```python
from build123d import *

# Parameters (mm, degrees)
BOSS_EXTRUDE1_DEPTH = 15
SKETCH4_R           = 1.5875
CUT_EXTRUDE2_DEPTH  = 25.005207768
SKETCH6_W           = 7.103151839
SKETCH6_H           = 13
SKETCH6_W_2         = 1.996848161
BOSS_EXTRUDE2_DEPTH = 8
SKETCH7_W           = 5.475
SKETCH7_H           = 24
CUT_EXTRUDE3_DEPTH  = 30.261749777


with BuildPart() as part:
    # Sketch1 → Boss-Extrude1 (new body)
    with BuildSketch(Plane(origin=(0, 0, 0), x_dir=(0, 0, -1), z_dir=(1, 0, 0))):
        with BuildLine():
            Line((6.5, 0), (13.5, 0))
            Line((13.5, 0), (13.5, -13))
            Line((13.5, -13), (-13.5, -13))
            Line((-13.5, -13), (-13.5, 0))
            Line((-13.5, 0), (-6.5, 0))
            ThreePointArc((-6.5, 0), (0, -6.5), (6.5, 0))
        make_face()
    extrude(amount=BOSS_EXTRUDE1_DEPTH)

    # Sketch4 → Cut-Extrude2 (cut, through all)
    with BuildSketch(Plane.XZ.offset(13)):
        with Locations(Location((10.2375, -10.75, 0), (0, 0, 270))):
            Circle(SKETCH4_R)
        with Locations(Location((10.2375, 10.75, 0), (0, 0, 270))):
            Circle(SKETCH4_R)
    extrude(amount=-CUT_EXTRUDE2_DEPTH, mode=Mode.SUBTRACT)

    # Sketch6 → Boss-Extrude2 (add)
    with BuildSketch(Plane.XY.offset(13.5)):
        with Locations((11.448424081, -6.5)):
            Rectangle(SKETCH6_W, SKETCH6_H)
        with Locations((0.998424081, -6.5)):
            Rectangle(SKETCH6_W_2, SKETCH6_H)
    extrude(amount=BOSS_EXTRUDE2_DEPTH)

    # Sketch7 → Cut-Extrude3 (cut, through all)
    with BuildSketch(Plane(origin=(0, 0, 0), x_dir=(1, 0, 0), z_dir=(0, 1, 0))):
        with Locations((2.7375, 1.5)):
            Rectangle(SKETCH7_W, SKETCH7_H)
    extrude(amount=-CUT_EXTRUDE3_DEPTH, mode=Mode.SUBTRACT)


solid = part.part
```
Part model, mm, in its own coordinate system. A direction names the side the tool comes from. Round coordinates to 2 decimals unless told otherwise and drop trailing zeros. Loops run counter-clockwise (first coordinate to the right, second up) from the corner with the lowest first, then second, coordinate; pieces in that order, holes last. Notation, with made-up numbers: (-36.75, -35) -> (-0.75, -35) arc R23 cw to (-0.75, 4) -> close; hole circle Ø4 at (-40, 85). An arc over 180 degrees is marked (long way). Use CSV: the item, a comma, the result in double quotes. Start each with the question number.
1) Which spindle directions (+Z, -Z, +X, -X, +Y, -Y) get a long thin tool onto all of the face, cutting with end or side? Do faces 1 (the cylindrical face through (10.2, -6.5, 0.1)), 2 (the flat face through (7.897, -7, 17)), 3 (the flat face through (3, -6, 10.5)). Say none if no direction does.
2) Drop flat-ended pins along their axis: P1, Ø6.5, axis at y = -4.5, z = -1.5, coming from the -X side (3 decimals); P2, Ø2.5, axis at x = 10.24, z = 10.75, coming from the -Y side. Give the stop position or say it passes through.
3) Cut at A-A, the plane z = 14.5. Write the cut outline in (x, y).
4) Pull direction Z, two halves, no side cores. Call faces 4 (the cylindrical face through (11.81, -6.59, -10.54)), 5 (the flat face through (5, -7, 13.5)), 6 (the flat face through (11, 0, -9)): +Z half, -Z half, draft (parallel to the pull), parting line (faces both ways), or undercut.
5) Wall check: L1, parallel to X at y = -3, z = 14; L2, parallel to X at y = -6.75, z = -10.75 (3 decimals); L3, parallel to Z at x = 3.25, y = -8.25. Give the ranges that are in metal, low to high. Write a range as [from, to].
6) Cut at B-B, the plane y = -4. Give the number of separate pieces and of enclosed holes in the cut face, plus the area to 3 significant figures.
7) Cut at C-C, the plane z = -10.75. Write the cut outline in (x, y) (3 decimals).
Determined:
1,face 1,"+X, -X, +Y"
1,face 2,"+Z, +Y, -Y"
1,face 3,"-Z, -X, +Y, -Y"
2,P1,"stops at x = 5.475"
2,P2,"passes through"
3,outline,"(0, -13) -> (2, -13) -> (2, 0) -> (0, 0) -> close; (7.9, -13) -> (15, -13) -> (15, 0) -> (7.9, 0) -> close"
4,face 4,"undercut"
4,face 5,"+Z half"
4,face 6,"draft"
5,L1,"x = [0, 2], [7.9, 15]"
5,L2,"x = [5.475, 8.65], [11.825, 15]"
5,L3,"z = [10.5, 13.5]"
6,separate pieces,"2"
6,enclosed holes,"2"
6,area,"233 mm2"
7,outline,"(5.475, -13) -> (8.65, -13) -> (8.65, 0) -> (5.475, 0) -> close; (11.825, -13) -> (15, -13) -> (15, 0) -> (11.825, 0) -> close"
